Here's how the part is built. I have some questions about the finished solid (model axes, mm). A direction names the side the tool comes from. Give positions to 0.01 mm unless a question says otherwise; leave off trailing zeros. Write each loop counter-clockwise with the first axis right and the second up, starting at its lowest first coordinate (ties: lowest second). Pieces come first, ordered by that corner, then holes. Notation, with made-up numbers: (6, 74) - (42, 74) arc R11 cw to (42, 88) - close; hole circle Ø9 at (8.25, 34). An arc over 180 degrees is marked (long way). Use a Markdown table: item, result.
```python
from build123d import *

# Parameters (mm, degrees)
F0_R      = 30
F1_DEPTH  = 10
F2_R      = 25.25
F3_DEPTH  = 5
F4_R      = 6.3
F5_DEPTH  = 10.001
F6_R      = 1.35
F7_DEPTH  = 10.001
F8_R      = 2.75
F9_DEPTH  = 5.001
F10_R     = 30
F10_R_2   = 20
F11_DEPTH = 5
F12_W     = 30
F12_H     = 24.7647633499
F13_DEPTH = 5
F14_R     = 13.25
F14_R_2   = 12.75
F14_R_3   = 6.75
F14_R_4   = 6.3
F15_DEPTH = 0.4


with BuildPart() as f1:
    # F0 (on Top) → F1 (new body)
    with BuildSketch(Plane.XY):
        Circle(F0_R)
    extrude(amount=F1_DEPTH)

    # F2 (on face) → F3 (cut)
    with BuildSketch(Plane.XY.offset(10)):
        Circle(F2_R)
    extrude(amount=-F3_DEPTH, mode=Mode.SUBTRACT)

    # F4 (on Top) → F5 (cut, through all)
    with BuildSketch(Plane.XY):
        Circle(F4_R)
    extrude(amount=F5_DEPTH, mode=Mode.SUBTRACT)

    # F6 (on face) → F7 (cut, through all)
    with BuildSketch(Plane.XY.offset(10)):
        with Locations((23.8156986041, 13.75)):
            Circle(F6_R)
        with Locations((0, -27.5)):
            Circle(F6_R)
        with Locations((-23.8156986041, 13.75)):
            Circle(F6_R)
    extrude(amount=-F7_DEPTH, mode=Mode.SUBTRACT)

    # F8 (on face) → F9 (cut, through all)
    with BuildSketch(Plane.XY.offset(5)):
        with Locations((0, 17)):
            Circle(F8_R)
    extrude(amount=-F9_DEPTH, mode=Mode.SUBTRACT)

    # F10 (on face) → F11 (join)
    with BuildSketch(Plane(origin=(0, 0, 0), x_dir=(1, 0, 0), z_dir=(0, 0, -1))):
        Circle(F10_R)
        Circle(F10_R_2, mode=Mode.SUBTRACT)
    extrude(amount=F11_DEPTH)

    # F12 (on Top) → F13 (cut)
    with BuildSketch(Plane.XY):
        with Locations((0, 20.9111002412)):
            Rectangle(F12_W, F12_H)
    extrude(amount=-F13_DEPTH, mode=Mode.SUBTRACT)

    # F14 (on face) → F15 (join)
    with BuildSketch(Plane.XY.offset(5)):
        Circle(F14_R)
        Circle(F14_R_2, mode=Mode.SUBTRACT)
        Circle(F14_R_3)
        Circle(F14_R_4, mode=Mode.SUBTRACT)
    extrude(amount=F15_DEPTH)


solid = f1.part
```
Item 1: I need wall thicknesses on line 1 along Y through (x, z) = (0, 6.6); line 2 along Z through (x, y) = (-4, -21); line 3 along Y through (x, z) = (17, 5.5). Which ranges of each line are inside material? Lowest first, please. Write a range as [from, to].
Values:
| item | result |
|---|---|
| line 1 | y = [-30, -28.85], [-26.15, -25.25], [25.25, 30] |
| line 2 | z = [-5, 5] |
| line 3 | y = [-24.72, -18.67], [18.67, 24.72] |
Item 2: If we section it at A-A, the plane y = 0: Write out the boundary of the cut face in (x, z).
Values:
| item | result |
|---|---|
| outline | (-30, -5) - (-20, -5) - (-20, 0) - (-6.3, 0) - (-6.3, 5.4) - (-6.75, 5.4) - (-6.75, 5) - (-12.75, 5) - (-12.75, 5.4) - (-13.25, 5.4) - (-13.25, 5) - (-25.25, 5) - (-25.25, 10) - (-30, 10) - close; (6.3, 0) - (20, 0) - (20, -5) - (30, -5) - (30, 10) - (25.25, 10) - (25.25, 5) - (13.25, 5) - (13.25, 5.4) - (12.75, 5.4) - (12.75, 5) - (6.75, 5) - (6.75, 5.4) - (6.3, 5.4) - close |
Item 3: If we section it at D-D, the plane x = 9: Write out the boundary of the cut face in (y, z), plus the area to 3 significant figures.
Values:
| item | result |
|---|---|
| outline | (-28.62, -5) - (-17.86, -5) - (-17.86, 0) - (28.62, 0) - (28.62, 10) - (23.59, 10) - (23.59, 5) - (9.72, 5) - (9.72, 5.4) - (9.03, 5.4) - (9.03, 5) - (-9.03, 5) - (-9.03, 5.4) - (-9.72, 5.4) - (-9.72, 5) - (-23.59, 5) - (-23.59, 10) - (-28.62, 10) - close |
| area | 391 mm2 |
Item 4: If we section it at B-B, the plane x = 0: Count the separate pieces of the cut face and the enclosed holes in it, plus the area to 3 significant figures.
Values:
| item | result |
|---|---|
| separate pieces | 3 |
| enclosed holes | 0 |
| area | 281 mm2 |
Item 5: Will these pins go through, and if not, where does the flat tip stop? pin 1 Ø8 at (x, z) = (14.5, 6.5) entering from +Y; pin 2 Ø8 at (x, y) = (23, 0) entering from +Z; pin 3 Ø0.8 at (x, y) = (0.5, -27.5) entering from +Z; pin 4 Ø2 at (x, y) = (16, 15) entering from +Z.
Values:
| item | result |
|---|---|
| pin 1 | stops at y = 28.1 |
| pin 2 | stops at z = 10 |
| pin 3 | stops at z = 0 |
| pin 4 | stops at z = 5 |
Item 6: If we section it at C-C, the plane z = 8.5: Write out the boundary of the cut face in (x, y), plus the area to 3 significant figures.
Values:
| item | result |
|---|---|
| outline | circle Ø60 at (0, 0); hole circle Ø50.5 at (0, 0); hole circle Ø2.7 at (-23.82, 13.75); hole circle Ø2.7 at (0, -27.5); hole circle Ø2.7 at (23.82, 13.75) |
| area | 807 mm2 |
Item 7: For faces 1 (the cylindrical face through (-5, -3.83, 2.66)), 2 (the cylindrical face through (-2.764, -12.447, 5.197)), 3 (the cylindrical face through (0.64, -19.99, -2.46)), 4 (the flat face through (-15, 20, -2)), 5 (the flat face through (0, -21, -5)), which set-ups out of +Z, -Z, +X, -X, +Y, -Y let a thin tool reach every point of the face, with its end or its side?
Values:
| item | result |
|---|---|
| face 1 | +Z, -Z |
| face 2 | +Z |
| face 3 | -Z |
| face 4 | -Z, +Y |
| face 5 | -Z, +X, -X, +Y, -Y |
Item 8: Thinking about a two-plate mould opening in X: for faces 6 (the cylindrical face through (-3.905, -29.745, 2.605)), 7 (the flat face through (-16, -20, 10)), 8 (the cylindrical face through (-5.47, -24.65, 7.54)), which applies, +X half, -X half, draft (parallel to the pull), parting line (faces both ways), or undercut?
Values:
| item | result |
|---|---|
| face 6 | parting line |
| face 7 | draft |
| face 8 | undercut |
